Geometry check sheet. Reference: the model listing, model coordinates, mm. Round coordinates to 2 decimals unless told otherwise and drop trailing zeros. Order: outer loops, then holes, each group sorted by start corner. A loop starts at its lowest first (then second) coordinate and runs counter-clockwise, first axis right, second up.
```python
from build123d import *

# Parameters (mm, degrees)
P_IDAT_VYSUNUT_M1_DEPTH  = 30
ODEBRAT_VYSUNUT_M1_DEPTH = 86.813751812
LINPOLE1_COUNT           = 3
LINPOLE1_PITCH           = 20
LINPOLE1_COUNT_DIR2      = 6
LINPOLE1_PITCH_DIR2      = 14
ZAOBLIT1_R               = 1


with BuildPart() as part:
    # Skica1 → Přidat vysunutím1 (new, symmetric)
    with BuildSketch(Plane.XY):
        Polygon((10, 0), (0, 0), (0, 80), (2, 80), (2, 4), (10, 4), align=None)
    extrude(amount=P_IDAT_VYSUNUT_M1_DEPTH, both=True)

    # Skica2 → Odebrat vysunutím1 (cut, through all)
    with BuildSketch(Plane(origin=(2, 0, 0), x_dir=(0, 0, -1), z_dir=(1, 0, 0))):
        with BuildLine():
            Line((-23.5, 16.5), (-16.5, 16.5))
            ThreePointArc((-16.5, 16.5), (-14, 14), (-16.5, 11.5))
            Line((-16.5, 11.5), (-23.5, 11.5))
            ThreePointArc((-23.5, 11.5), (-26, 14), (-23.5, 16.5))
        make_face()
    odebrat_vysunut_m1 = extrude(amount=-ODEBRAT_VYSUNUT_M1_DEPTH, mode=Mode.SUBTRACT)

    # LinPole1: Odebrat vysunut_m1 3 × 6
    with Locations(*[(0, j * LINPOLE1_PITCH_DIR2, -i * LINPOLE1_PITCH) for i in range(LINPOLE1_COUNT) for j in range(LINPOLE1_COUNT_DIR2) if (i, j) != (0, 0)]):
        add(odebrat_vysunut_m1, mode=Mode.SUBTRACT)

    # Zaoblit1
    zaoblit1_edges = [part.edges().sort_by_distance(p)[0] for p in [
        (1, 80, 30),
        (10, 2, 30),
        (1, 80, -30),
        (10, 2, -30),
    ]]
    fillet(zaoblit1_edges, radius=ZAOBLIT1_R)


solid = part.part
```
(1) Draft check along Y on faces 1 (the flat face through (2, 43, 7)), 2 (the flat face through (1, 58.5, -20)). Enter one of: released by +Y, released by -Y, zero draft, split by the parting line, or undercut.
Returned:
face 1: zero draft
face 2: undercut
(2) Sectioned sample at D-D, the plane z = 13. Record the cut outline in (x, y).
Returned:
outline: (0, 0) - (10, 0) - (10, 4) - (2, 4) - (2, 80) - (0, 80) - close
(3) Sectioned sample at B-B, the plane z = -15. Record the cut outline in (x, y).
Returned:
outline: (0, 0) - (10, 0) - (10, 4) - (2, 4) - (2, 12) - (0, 12) - close; (0, 16) - (2, 16) - (2, 26) - (0, 26) - close; (0, 30) - (2, 30) - (2, 40) - (0, 40) - close; (0, 44) - (2, 44) - (2, 54) - (0, 54) - close; (0, 58) - (2, 58) - (2, 68) - (0, 68) - close; (0, 72) - (2, 72) - (2, 80) - (0, 80) - close
(4) Material ranges on line 1 (Y direction, x = 1.5, z = -18); line 2 (X direction, y = 25, z = -4.5); line 3 (Y direction, x = 8.25, z = 19), recorded low to high.
Returned:
line 1: y = 0 to 11.5, 16.5 to 25.5, 30.5 to 39.5, 44.5 to 53.5, 58.5 to 67.5, 72.5 to 80
line 2: x = 0 to 2
line 3: y = 0 to 4
(5) Sectioned sample at A-A, the plane y = 70. Record the cut outline in (x, z), and give its area (3 significant figures).
Returned:
outline: (0, -30) - (2, -30) - (2, -26) - (0, -26) - close; (0, -14) - (2, -14) - (2, -6) - (0, -6) - close; (0, 6) - (2, 6) - (2, 14) - (0, 14) - close; (0, 26) - (2, 26) - (2, 30) - (0, 30) - close
area: 48.0 mm2
(6) Depth check by flat-ended pin: P1, Ø5, axis at x = 7, z = -13, coming from the +Y side; P2, Ø12, axis at y = 41.5, z = -8, coming from the +X side. Enter the tip coordinate at first touch or a pass-through.
Returned:
P1: stops at y = 4
P2: stops at x = 2
(7) Sectioned sample at C-C, the plane x = 1. Give the number of separate pieces and of enclosed holes in the cut face, and give its area (3 significant figures).
Returned:
separate pieces: 1
enclosed holes: 15
area: 3,980 mm2
